For this review, take the finished solid that the model builds, in its own axes (mm). Round coordinates to 2 decimals unless told otherwise and drop trailing zeros. Write each loop counter-clockwise with the first axis right and the second up, starting at its lowest first coordinate (ties: lowest second). Pieces come first, ordered by that corner, then holes. Notation, with made-up numbers: M 70,70.25 L 97,70.25 A20 ccw 97,75.25 Z; hole C 37.25,18.25 d1. An arc over 180 degrees is marked long. Answer in a Markdown table with one row per item.
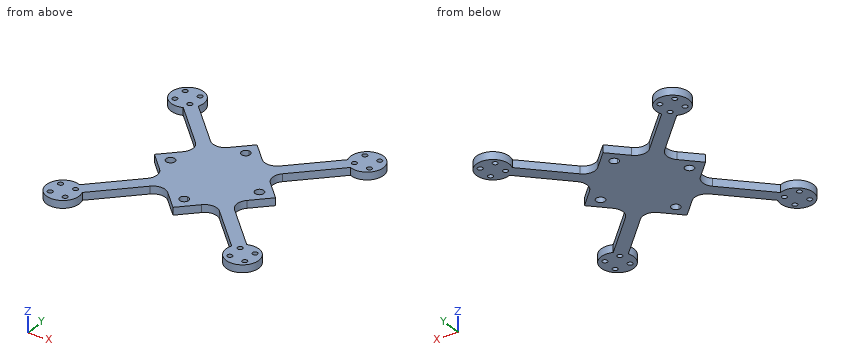
```python
from build123d import *

# Parameters (mm, degrees)
SKETCH_R  = 1
PAD_DEPTH = 3
FILLET_R  = 5


with BuildPart() as part:
    # Sketch → Pad (new body)
    with BuildSketch(Plane.XY):
        with BuildLine():
            ThreePointArc((-29.698485, 33.234019), (-40.305087, 40.305087), (-33.234019, 29.698485))
            Line((-33.234019, 29.698485), (-13.810747, 10.275213))
            Line((-13.810747, 10.275213), (-24.08596, 0))
            Line((-13.810747, -10.275213), (-24.08596, 0))
            Line((-33.234019, -29.698485), (-13.810747, -10.275213))
            ThreePointArc((-33.234019, -29.698485), (-40.305087, -40.305087), (-29.698485, -33.234019))
            Line((-29.698485, -33.234019), (-10.275213, -13.810747))
            Line((0, -24.08596), (-10.275213, -13.810747))
            Line((0, -24.08596), (10.275213, -13.810747))
            Line((29.698485, -33.234019), (10.275213, -13.810747))
            ThreePointArc((29.698485, -33.234019), (40.305087, -40.305087), (33.234019, -29.698485))
            Line((33.234019, -29.698485), (13.810747, -10.275213))
            Line((13.810747, -10.275213), (24.08596, 0))
            Line((13.810747, 10.275213), (24.08596, 0))
            Line((33.234019, 29.698485), (13.810747, 10.275213))
            ThreePointArc((33.234019, 29.698485), (40.305087, 40.305087), (29.698485, 33.234019))
            Line((29.698485, 33.234019), (10.275213, 13.810747))
            Line((0, 24.08596), (10.275213, 13.810747))
            Line((0, 24.08596), (-10.275213, 13.810747))
            Line((-29.698485, 33.234019), (-10.275213, 13.810747))
        make_face()
        with Locations((-38.678741, 38.678741)):
            Circle(SKETCH_R, mode=Mode.SUBTRACT)
        with Locations((-38.678741, 32.739044)):
            Circle(SKETCH_R, mode=Mode.SUBTRACT)
        with Locations((-32.739044, 38.678741)):
            Circle(SKETCH_R, mode=Mode.SUBTRACT)
        with Locations((-32.739044, 32.739044)):
            Circle(SKETCH_R, mode=Mode.SUBTRACT)
        with Locations((38.678741, -38.678741)):
            Circle(SKETCH_R, mode=Mode.SUBTRACT)
        with Locations((38.678741, -32.739044)):
            Circle(SKETCH_R, mode=Mode.SUBTRACT)
        with Locations((32.739044, -38.678741)):
            Circle(SKETCH_R, mode=Mode.SUBTRACT)
        with Locations((32.739044, -32.739044)):
            Circle(SKETCH_R, mode=Mode.SUBTRACT)
        with Locations((-38.678741, -38.678741)):
            Circle(SKETCH_R, mode=Mode.SUBTRACT)
        with Locations((-38.678741, -32.739044)):
            Circle(SKETCH_R, mode=Mode.SUBTRACT)
        with Locations((-32.739044, -38.678741)):
            Circle(SKETCH_R, mode=Mode.SUBTRACT)
        with Locations((-32.739044, -32.739044)):
            Circle(SKETCH_R, mode=Mode.SUBTRACT)
        with Locations((38.678741, 38.678741)):
            Circle(SKETCH_R, mode=Mode.SUBTRACT)
        with Locations((38.678741, 32.739044)):
            Circle(SKETCH_R, mode=Mode.SUBTRACT)
        with Locations((32.739044, 38.678741)):
            Circle(SKETCH_R, mode=Mode.SUBTRACT)
        with Locations((32.739044, 32.739044)):
            Circle(SKETCH_R, mode=Mode.SUBTRACT)
        with BuildLine():
            ThreePointArc((-0.002953, 19.427669), (-1.74985, 17.700664), (-0.048936, 15.928353))
            ThreePointArc((-0.048936, 15.928353), (1.74985, 17.654676), (-0.002953, 19.427669))
        make_face(mode=Mode.SUBTRACT)
        with BuildLine():
            ThreePointArc((-15.92767, 0), (-17.67767, 1.75), (-19.42767, 0))
            ThreePointArc((-19.42767, 0), (-17.67767, -1.75), (-15.92767, 0))
        make_face(mode=Mode.SUBTRACT)
        with BuildLine():
            ThreePointArc((0.002953, -19.427669), (1.74985, -17.700664), (0.048936, -15.928353))
            ThreePointArc((0.048936, -15.928353), (-1.74985, -17.654676), (0.002953, -19.427669))
        make_face(mode=Mode.SUBTRACT)
        with BuildLine():
            ThreePointArc((15.92767, 0), (17.67767, -1.75), (19.42767, 0))
            ThreePointArc((19.42767, 0), (17.67767, 1.75), (15.92767, 0))
        make_face(mode=Mode.SUBTRACT)
    extrude(amount=PAD_DEPTH)

    # Fillet
    fillet_edges = [part.edges().sort_by_distance(p)[0] for p in [
        (13.810747, 10.275213, 1.5),
        (13.810747, -10.275213, 1.5),
        (-10.275213, -13.810747, 1.5),
        (-13.810747, 10.275213, 1.5),
        (10.275213, 13.810747, 1.5),
        (-10.275213, 13.810747, 1.5),
        (-13.810747, -10.275213, 1.5),
        (10.275213, -13.810747, 1.5),
    ]]
    fillet(fillet_edges, radius=FILLET_R)


solid = part.part
```
Q1. For probe 1 along Y at (x, z) = (16.5, 1.1); probe 2 along X at (y, z) = (19, 0.7); probe 3 along X at (y, z) = (-1, 2.8), list the stretches that pass through material, from the lowest coordinate up.
Found:
| item | result |
|---|---|
| probe 1 | -20.04 to -12.68, -7.87 to -1.29, 1.29 to 7.87, 12.68 to 20.04 |
| probe 2 | -22.54 to -15.46, -5.09 to -1.15, 1.15 to 5.09, 15.46 to 22.54 |
| probe 3 | -23.09 to -19.11, -16.24 to 16.24, 19.11 to 23.09 |
Q2. Insertion check: P1, Ø2.5, axis at x = 38.68, y = -32.74, coming from the -Z side; P2, Ø1.8, axis at x = -38.68, y = -32.74, coming from the +Z side. Each pin has a flat end and moves straight along its axis. Give the tip position at first contact, or say it passes through.
Found:
| item | result |
|---|---|
| P1 | z = 0 |
| P2 | through |
Q3. Take a section at B-B (z = 1.75). State how many separate pieces and enclosed holes the cut face has, then the cut area to 3 significant figures.
Found:
| item | result |
|---|---|
| separate pieces | 1 |
| enclosed holes | 20 |
| area | 2,190 mm² |
Q4. Take a section at D-D (x = -4.5). State the section outline as (y, z) points.
Found:
| item | result |
|---|---|
| outline | M -19.59,0 L 19.59,0 L 19.59,3 L -19.59,3 Z |
Q5. Take a section at A-A (y = -35). State the section outline as (x, z) points, then the cut area to 3 significant figures.
Found:
| item | result |
|---|---|
| outline | M -42.17,0 L -29.25,0 L -29.25,3 L -42.17,3 Z; M 29.25,0 L 42.17,0 L 42.17,3 L 29.25,3 Z |
| area | 77.5 mm² |
Q6. Take a section at C-C (y = 5.5). State the section outline as (x, z) points, then the cut area to 3 significant figures.
Found:
| item | result |
|---|---|
| outline | M -18.59,0 L 18.59,0 L 18.59,3 L -18.59,3 Z |
| area | 112 mm² |
